The model under review builds one solid part; all positions refer to its coordinate system, in mm. A direction names the side the tool comes from. Give positions to 0.01 mm unless a question says otherwise; leave off trailing zeros. Order: outer loops, then holes, each group sorted by start corner. A loop starts at its lowest first (then second) coordinate and runs counter-clockwise, first axis right, second up. Notation, with made-up numbers: (-24.5, 22.5) - (-9.5, 22.5) arc R22 ccw to (-9.5, 40.5) - close; hole circle Ø5 at (-15.5, -30). An arc over 180 degrees is marked (long way). Use CSV: the item, a comma, the result in double quotes. Start each with the question number.
```python
from build123d import *

# Parameters (mm, degrees)
BASE_FLANGE1_DEPTH = 482.6
SKETCH2_R          = 2.45745
CUT_EXTRUDE1_DEPTH = 3.175
SKETCH3_R          = 2.45745
SKETCH3_R_2        = 4.7625
CUT_EXTRUDE2_DEPTH = 3.175
SKETCH4_R          = 2.45745
CUT_EXTRUDE3_DEPTH = 3.175
FILLET1_R          = 3.175


# Sheet-metal steps are written as plain solids
with BuildPart() as part:
    # Sketch1 → Base-Flange1 (new body)
    with BuildSketch(Plane(origin=(0, 0, 0), x_dir=(1, 0, 0), z_dir=(0, 1, 0))):
        with BuildLine():
            Line((0, 177.8), (0, 6.35))
            ThreePointArc((0, 6.35), (1.859871939, 1.859871939), (6.35, 0))
            Line((6.35, 0), (66.675, 0))
            ThreePointArc((66.675, 0), (71.165128061, 1.859871939), (73.025, 6.35))
            Line((73.025, 6.35), (73.025, 50.8))
            Line((73.025, 50.8), (69.85, 50.8))
            Line((69.85, 50.8), (69.85, 6.35))
            ThreePointArc((69.85, 6.35), (68.92006403, 4.10493597), (66.675, 3.175))
            Line((66.675, 3.175), (6.35, 3.175))
            ThreePointArc((6.35, 3.175), (4.10493597, 4.10493597), (3.175, 6.35))
            Line((3.175, 6.35), (3.175, 177.8))
            Line((3.175, 177.8), (0, 177.8))
        make_face()
    extrude(amount=BASE_FLANGE1_DEPTH)

    # Sketch2 → Cut-Extrude1 (cut)
    with BuildSketch(Plane(origin=(73.025, 0, 0), x_dir=(0, 0, -1), z_dir=(1, 0, 0))):
        with Locations((12.7, 457.2)):
            Circle(SKETCH2_R)
        with Locations((44.45, 457.2)):
            Circle(SKETCH2_R)
        with Locations((12.7, 25.4)):
            Circle(SKETCH2_R)
        with Locations((44.45, 25.4)):
            Circle(SKETCH2_R)
        with Locations((44.45, 241.3)):
            Circle(SKETCH2_R)
        with Locations((12.7, 241.3)):
            Circle(SKETCH2_R)
        with BuildLine():
            Line((31.9484375, 423.8625), (31.9484375, 414.3375))
            ThreePointArc((31.9484375, 414.3375), (28.575, 410.9640625), (25.2015625, 414.3375))
            Line((25.2015625, 414.3375), (25.2015625, 423.8625))
            ThreePointArc((25.2015625, 423.8625), (28.575, 427.2359375), (31.9484375, 423.8625))
        make_face()
        with BuildLine():
            Line((31.9484375, 68.2625), (31.9484375, 58.7375))
            ThreePointArc((31.9484375, 58.7375), (28.575, 55.3640625), (25.2015625, 58.7375))
            Line((25.2015625, 58.7375), (25.2015625, 68.2625))
            ThreePointArc((25.2015625, 68.2625), (28.575, 71.6359375), (31.9484375, 68.2625))
        make_face()
    extrude(amount=-CUT_EXTRUDE1_DEPTH, mode=Mode.SUBTRACT)

    # Sketch3 → Cut-Extrude2 (cut)
    with BuildSketch(Plane.ZY):
        with Locations((-165.1, 457.2)):
            Circle(SKETCH3_R)
        with Locations((-165.1, 25.4)):
            Circle(SKETCH3_R)
        with Locations((-165.1, 241.3)):
            Circle(SKETCH3_R)
        with Locations((-114.3, 25.4)):
            Circle(SKETCH3_R)
        with Locations((-114.3, 241.3)):
            Circle(SKETCH3_R)
        with Locations((-114.3, 457.2)):
            Circle(SKETCH3_R)
        with Locations((-63.5, 25.4)):
            Circle(SKETCH3_R)
        with Locations((-63.5, 241.3)):
            Circle(SKETCH3_R)
        with Locations((-63.5, 457.2)):
            Circle(SKETCH3_R)
        with Locations((-139.7, 457.2)):
            Circle(SKETCH3_R_2)
        with Locations((-139.7, 25.4)):
            Circle(SKETCH3_R_2)
    extrude(amount=-CUT_EXTRUDE2_DEPTH, mode=Mode.SUBTRACT)

    # Sketch4 → Cut-Extrude3 (cut)
    with BuildSketch(Plane.XY):
        with Locations((12.7, 457.2)):
            Circle(SKETCH4_R)
        with Locations((12.7, 241.3)):
            Circle(SKETCH4_R)
        with Locations((12.7, 25.4)):
            Circle(SKETCH4_R)
    extrude(amount=-CUT_EXTRUDE3_DEPTH, mode=Mode.SUBTRACT)

    # Fillet1
    fillet1_edges = [part.edges().sort_by_distance(p)[0] for p in [
        (1.5875, 0, -177.8),
        (71.4375, 0, -50.8),
        (1.5875, 482.6, -177.8),
        (71.4375, 482.6, -50.8),
    ]]
    fillet(fillet1_edges, radius=FILLET1_R)


solid = part.part
```
1. To check wall thickness, follow L1, parallel to Y at x = 1, z = -114; L2, parallel to Y at x = 1.85, z = -165.1; L3, parallel to Z at x = 2, y = 25. State the ranges of each line that lie inside material, in increasing order. Write a range as [from, to].
2. Clearance check with flat-ended pins moving along their axes: pin 1 (5.5 mm diameter, centred on y = 241.3, z = -63.5, fed in from -X); pin 2 (1.6 mm diameter, centred on x = 71, y = 62, fed in from +Z); pin 3 (8.5 mm diameter, centred on y = 457.2, z = -139.7, fed in from -X); pin 4 (8 mm diameter, centred on y = 25.4, z = -63.5, fed in from +X) (3 decimals). State where each tip first meets the part, or that it passes through.
3. Mouldability with a two-part tool opening along Y and no side actions: class faces 3 (the face through (1, 482.6, -68)), 4 (the face through (1.57, 455.38, -135.3)), 5 (the face through (1.565, 26.831, -135.157)), 6 (the face through (1, 0, -68)) as pulls with the +Y half, pulls with the -Y half, needs draft (parallel to the pull), parting line crosses it, or undercut.
4. Consider section C-C (x = 59). Give the boundary of the cut face in (y, z) (3 decimals).
5. Consider section A-A (z = -139.7). Give the boundary of the cut face in (x, y) (1 decimal), and give its area (3 significant figures).
6. Consider section B-B (y = 353). Give the boundary of the cut face in (x, z) (3 decimals), and give its area (3 significant figures).
7. Tool access review of faces 1 (the face through (0, 238, -93)), 2 (the face through (69.85, 238, -29)): name each direction out of +Z, -Z, +X, -X, +Y, -Y from which nothing blocks a thin tool from reaching the whole face with its end or side.
8. Consider section D-D (z = -121). Give the boundary of the cut face in (x, y) (3 decimals).
Answers follow:
1,L1,"y = [0, 22.96], [27.84, 238.86], [243.74, 454.76], [459.64, 482.6]"
1,L2,"y = [0, 22.94], [27.86, 238.84], [243.76, 454.74], [459.66, 482.6]"
1,L3,"z = [-177.8, -167.52], [-162.68, -144.45], [-134.95, -116.72], [-111.88, -65.92], [-61.08, -1.72]"
2,pin 1,"stops at x = 0"
2,pin 2,"stops at z = -1.07"
2,pin 3,"passes through"
2,pin 4,"stops at x = 3.175"
3,face 3,"pulls with the +Y half"
3,face 4,"undercut"
3,face 5,"undercut"
3,face 6,"pulls with the -Y half"
4,outline,"(0, -3.175) - (482.6, -3.175) - (482.6, 0) - (0, 0) - close"
5,outline,"(0, 0) - (3.2, 0) - (3.2, 20.6) - (0, 20.6) - close; (0, 30.2) - (3.2, 30.2) - (3.2, 452.4) - (0, 452.4) - close; (0, 462) - (3.2, 462) - (3.2, 482.6) - (0, 482.6) - close"
5,area,"1,470 mm^2"
6,outline,"(0, -177.8) - (3.175, -177.8) - (3.175, -6.35) arc R3.175 cw to (6.35, -3.175) - (66.675, -3.175) arc R3.175 cw to (69.85, -6.35) - (69.85, -50.8) - (73.025, -50.8) - (73.025, -6.35) arc R6.35 ccw to (66.675, 0) - (6.35, 0) arc R6.35 ccw to (0, -6.35) - close"
6,area,"925 mm^2"
7,face 1,"+Z, -Z, -X, +Y, -Y"
7,face 2,"-Z, +Y, -Y"
8,outline,"(0, 0) - (3.175, 0) - (3.175, 482.6) - (0, 482.6) - close"
